Work out the finished part from the listing and answer in its coordinate system (mm). A direction names the side the tool comes from. Coordinates: 2 decimals unless noted, no trailing zeros. Write each loop counter-clockwise with the first axis right and the second up, starting at its lowest first coordinate (ties: lowest second). Pieces come first, ordered by that corner, then holes. Notation, with made-up numbers: (52.25, -38) - (64.25, -38) arc R28 ccw to (64.25, -11) - close; hole circle Ø11 at (25.5, 89.25). An arc over 180 degrees is marked (long way). Use CSV: the item, a comma, the result in double quotes. Start each with the question number.
from build123d import *

# Parameters (mm, degrees)
MAIN_DEPTH                     = 20
SKETCH2_R                      = 3.1
SHAFTHOLE_DEPTH                = 5
SKETCH3_W                      = 10
SKETCH3_H                      = 10
MAKERBEAMRECTANGULARHOLE_DEPTH = 7
SKETCH4_R                      = 1.5
MAKERBEAMHOLE_DEPTH            = 9
FILLET1_R                      = 1


with BuildPart() as part:
    # Sketch1 → Main (new body)
    with BuildSketch(Plane.XY):
        with BuildLine():
            Line((-8, 5), (-8, 1.45))
            Line((-8, 1.45), (-9, 1.45))
            Line((-9, 1.45), (-9, -1.45))
            Line((-9, -1.45), (-8, -1.45))
            Line((-8, -1.45), (-8, -5))
            Line((-8, -5), (0, -5))
            ThreePointArc((0, -5), (5, 0), (0, 5))
            Line((0, 5), (-8, 5))
        make_face()
    extrude(amount=MAIN_DEPTH)

    # Sketch2 → ShaftHole (cut)
    with BuildSketch(Plane.XY.offset(20)):
        Circle(SKETCH2_R)
    extrude(amount=-SHAFTHOLE_DEPTH, mode=Mode.SUBTRACT)

    # Sketch3 → MakerBeamRectangularHole (cut, through all)
    with BuildSketch(Plane(origin=(-1, 0, 0), x_dir=(0, 0, -1), z_dir=(1, 0, 0))):
        with Locations((-5, 0)):
            Rectangle(SKETCH3_W, SKETCH3_H)
    extrude(amount=MAKERBEAMRECTANGULARHOLE_DEPTH, mode=Mode.SUBTRACT)

    # Sketch4 → MakerBeamHole (cut, through all)
    with BuildSketch(Plane(origin=(-1, 0, 0), x_dir=(0, 0, -1), z_dir=(1, 0, 0))):
        with Locations((-5, 0)):
            Circle(SKETCH4_R)
    extrude(amount=-MAKERBEAMHOLE_DEPTH, mode=Mode.SUBTRACT)

    # Fillet1
    fillet1_edges = [part.edges().sort_by_distance(p)[0] for p in [
        (-1, 0, 10),
    ]]
    fillet(fillet1_edges, radius=FILLET1_R)


solid = part.part
Item 1: Which of the six approach directions +Z, -Z, +X, -X, +Y, -Y give full straight-line access (tool end or side, diameter ignored) to faces 1 (the face through (-8.5, 1.45, 12.6)), 2 (the face through (-4, 5, 10)), 3 (the face through (-8.5, -1.45, 2.3)), 4 (the face through (0, 0, 15)), 5 (the face through (2, 0, 10))?
Item 2: A cutting plane is placed at B-B (x = -4.25). Determine the outline of the cut face in (y, z), then the cut area to 3 significant figures.
Item 3: Each of these flat-tipped pins is pushed along its axis until it touches: pin 1 (1.5 mm diameter, centred on x = 2, y = -0.5, fed in from -Z); pin 2 (1.8 mm diameter, centred on y = 3, z = 13.5, fed in from -X); pin 3 (5 mm diameter, centred on y = 0, z = 5, fed in from +X). Where does it stop, or does it pass through?
Item 4: A cutting plane is placed at D-D (z = 14.5). Determine the outline of the cut face in (x, y).
Item 5: Straight lines are drawn through the part: probe 1 along Y at (x, z) = (0, 17.9); probe 2 along Y at (x, z) = (-4, 5); probe 3 along Z at (x, y) = (2.75, -4). For each, find the intervals that lie inside material, in ascending order. Write a range as [from, to].
Item 6: Determine the mould class of faces 6 (the face through (1.43, -2.75, 17.54)), 7 (the face through (-8, 3, 10)), 8 (the face through (-8.5, -1.45, 12.6)) for opening direction X: +X half, -X half, draft (parallel to the pull), parting line (faces both ways), or undercut.
Item 7: A cutting plane is placed at A-A (z = 5). Determine the outline of the cut face in (x, y), then the cut area to 3 significant figures.
Item 8: A cutting plane is placed at C-C (y = 0). Determine the outline of the cut face in (x, z).
Calculated:
1,face 1,"+Z, -Z, -X, +Y"
1,face 2,"+Z, -Z, +X, -X, +Y"
1,face 3,"+Z, -Z, -X, -Y"
1,face 4,"+Z"
1,face 5,"-Z, +X, +Y, -Y"
2,outline,"(-5, 0) - (5, 0) - (5, 20) - (-5, 20) - close; hole circle Ø3 at (0, 5)"
2,area,"193 mm²"
3,pin 1,"stops at z = 10"
3,pin 2,"stops at x = -8"
3,pin 3,"stops at x = -1"
4,outline,"(-9, -1.45) - (-8, -1.45) - (-8, -5) - (0, -5) arc R5 ccw to (0, 5) - (-8, 5) - (-8, 1.45) - (-9, 1.45) - close"
5,probe 1,"y = [-5, -3.1], [3.1, 5]"
5,probe 2,"y = [-5, -1.5], [1.5, 5]"
5,probe 3,"z = [10, 20]"
6,face 6,"undercut"
6,face 7,"-X half"
6,face 8,"draft"
7,outline,"(-8, -5) - (-1, -5) - (-1, -1.5) - (-8, -1.5) - close; (-8, 1.5) - (-1, 1.5) - (-1, 5) - (-8, 5) - close"
7,area,"49.0 mm²"
8,outline,"(-9, 0) - (-1, 0) - (-1, 3.5) - (-9, 3.5) - close; (-9, 6.5) - (-1, 6.5) - (-1, 9) arc R1 cw to (0, 10) - (5, 10) - (5, 20) - (3.1, 20) - (3.1, 15) - (-3.1, 15) - (-3.1, 20) - (-9, 20) - close"
